Autodesk Inventor part; units mm, degrees
ref_plane "YZ Plane" through (0, 0, 0) normal (1, 0, 0) x (0, 1, 0)
ref_plane "XZ Plane" through (0, 0, 0) normal (0, 1, 0) x (-1, 0, 0)
ref_plane "XY Plane" through (0, 0, 0) normal (0, 0, 1) x (1, 0, 0)
sketch "Sketch1" plane through (0, 0, 0) normal (0, 1, 0) x (-1, 0, 0)
  line L0 (0, 0) -> (279.4, 0)
  line L1 (279.4, 0) -> (279.4, 53.34)
  line L2 (279.4, 53.34) -> (0, 53.34)
  line L3 (0, 53.34) -> (0, 0)
extrude "Extrusion1" add sketch "Sketch1" along normal blind 12.7
sketch "Sketch2" plane through (0, 12.7, 0) normal (0, 1, 0) x (1, 0, 0)
  line L0 (-12.7, -46.99) -> (-53.34, -46.99)
  line L1 (-53.34, -46.99) -> (-53.34, -6.35)
  line L2 (-53.34, -6.35) -> (-12.7, -6.35)
  line L3 (-12.7, -6.35) -> (-12.7, -46.99)
  line L4 (-279.4, -53.34) -> (0, -53.34)
  line L5 (0, -53.34) -> (0, 0)
  line L6 (-66.04, -46.99) -> (-106.68, -46.99)
  line L7 (-106.68, -46.99) -> (-106.68, -6.35)
  line L8 (-106.68, -6.35) -> (-66.04, -6.35)
  line L9 (-66.04, -6.35) -> (-66.04, -46.99)
  line L10 (-119.38, -46.99) -> (-160.02, -46.99)
  line L11 (-160.02, -46.99) -> (-160.02, -6.35)
  line L12 (-160.02, -6.35) -> (-119.38, -6.35)
  line L13 (-119.38, -6.35) -> (-119.38, -46.99)
  line L14 (-172.72, -46.99) -> (-213.36, -46.99)
  line L15 (-213.36, -46.99) -> (-213.36, -6.35)
  line L16 (-213.36, -6.35) -> (-172.72, -6.35)
  line L17 (-172.72, -6.35) -> (-172.72, -46.99)
  line L18 (-226.06, -46.99) -> (-266.7, -46.99)
  line L19 (-266.7, -46.99) -> (-266.7, -6.35)
  line L20 (-266.7, -6.35) -> (-226.06, -6.35)
  line L21 (-226.06, -6.35) -> (-226.06, -46.99)
  dimension "d2" = 40.64
  dimension "d3" = 40.64
  dimension "d4" = 6.35
  dimension "d5" = 12.7
  dimension "d6" = 40.64
  dimension "d7" = 12.7
  dimension "d8" = 40.64
  dimension "d9" = 12.7
  dimension "d10" = 40.64
  dimension "d11" = 12.7
  dimension "d12" = 40.64
  dimension "d13" = 12.7
extrude "Extrusion2" cut sketch "Sketch2" against normal through all
properties part number "Slide"
The model under review builds one solid part; all positions refer to its coordinate system, in mm. A direction names the side the tool comes from. Round coordinates to 2 decimals unless told otherwise and drop trailing zeros. Write each loop counter-clockwise with the first axis right and the second up, starting at its lowest first coordinate (ties: lowest second). Pieces come first, ordered by that corner, then holes.
(1) We need section C-C on y = 4.5. Give the boundary of the cut face in (x, z), and give its area (3 significant figures).
(2) Wall thickness on L1, parallel to X at y = 3.75, z = 38.5; L2, parallel to Z at x = -260, y = 9.75: over which ranges is each line inside the solid? List them lowest first.
(3) Machinability: for faces 4 (the flat face through (-140, 6, 6.35)), 5 (the flat face through (-142, 6, 53.34)), which of the approach directions +Z, -Z, +X, -X, +Y, -Y give a long, thin tool a straight path to every point of the face, cutting with its end or side? Answer none if there is none.
(4) We need section B-B on z = 25. Give the boundary of the cut face in (x, y), and give its area (3 significant figures).
(5) We need section A-A on x = -136. Give the boundary of the cut face in (y, z).
(6) Mouldability with a two-part tool opening along Z and no side actions: class faces 1 (the flat face through (-12.7, 6, 26)), 2 (the flat face through (-138, 0, 3)), 3 (the flat face through (-138, 6, 0)) as +Z half, -Z half, draft (parallel to the pull), parting line (faces both ways), or undercut.
Findings below:
1. outline: (-279.4, 0) - (0, 0) - (0, 53.34) - (-279.4, 53.34) - close; hole (-266.7, 6.35) - (-226.06, 6.35) - (-226.06, 46.99) - (-266.7, 46.99) - close; hole (-213.36, 6.35) - (-172.72, 6.35) - (-172.72, 46.99) - (-213.36, 46.99) - close; hole (-160.02, 6.35) - (-119.38, 6.35) - (-119.38, 46.99) - (-160.02, 46.99) - close; hole (-106.68, 6.35) - (-66.04, 6.35) - (-66.04, 46.99) - (-106.68, 46.99) - close; hole (-53.34, 6.35) - (-12.7, 6.35) - (-12.7, 46.99) - (-53.34, 46.99) - close
1. area: 6,650 mm2
2. L1: x = -279.4 to -266.7, -226.06 to -213.36, -172.72 to -160.02, -119.38 to -106.68, -66.04 to -53.34, -12.7 to 0
2. L2: z = 0 to 6.35, 46.99 to 53.34
3. face 4: +Y, -Y
3. face 5: +Z, +X, -X, +Y, -Y
4. outline: (-279.4, 0) - (-266.7, 0) - (-266.7, 12.7) - (-279.4, 12.7) - close; (-226.06, 0) - (-213.36, 0) - (-213.36, 12.7) - (-226.06, 12.7) - close; (-172.72, 0) - (-160.02, 0) - (-160.02, 12.7) - (-172.72, 12.7) - close; (-119.38, 0) - (-106.68, 0) - (-106.68, 12.7) - (-119.38, 12.7) - close; (-66.04, 0) - (-53.34, 0) - (-53.34, 12.7) - (-66.04, 12.7) - close; (-12.7, 0) - (0, 0) - (0, 12.7) - (-12.7, 12.7) - close
4. area: 968 mm2
5. outline: (0, 0) - (12.7, 0) - (12.7, 6.35) - (0, 6.35) - close; (0, 46.99) - (12.7, 46.99) - (12.7, 53.34) - (0, 53.34) - close
6. face 1: undercut
6. face 2: draft
6. face 3: -Z half
